Input: dimensioned drawing with shaded views. Units: mm. Origin: part minimum x, y, z. Give positions to 0.01 mm unless a question says otherwise; leave off trailing zeros. Loops run counter-clockwise (first coordinate to the right, second up) from the corner with the lowest first, then second, coordinate; pieces in that order, holes last.
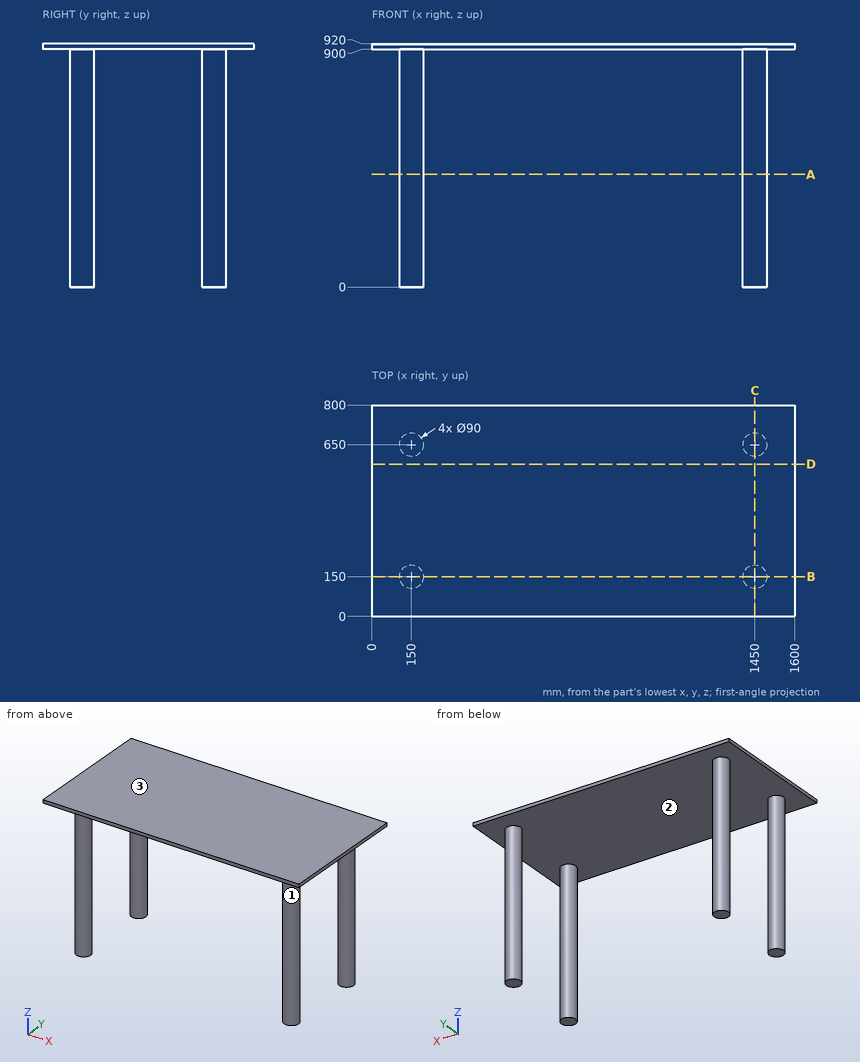
Item 1: Section query D-D on y = 576. Return loops of the section in (x, z), plus the area to 3 significant figures.
Values follow:
outline: (0, 900) - (1600, 900) - (1600, 920) - (0, 920) - close
area: 32,000 mm2
Item 2: Pin query (flat end, axial travel): pin 1 (5 mm diameter, centred on x = 468.5, y = 608.5, fed in from -Z). Return the tip coordinate at first contact, or that it passes through.
Values follow:
pin 1: stops at z = 900
Item 3: Section query B-B on y = 150. Return loops of the section in (x, z).
Values follow:
outline: (0, 900) - (105, 900) - (105, 0) - (195, 0) - (195, 900) - (1405, 900) - (1405, 0) - (1495, 0) - (1495, 900) - (1600, 900) - (1600, 920) - (0, 920) - close
Item 4: Ray query, probe 1 along Z at (x, y) = (194.5, 252.5); probe 2 along Y at (x, z) = (122.5, 771.5); probe 3 along X at (y, z) = (176.5, 828). Return the intervals inside material, ascending.
Values follow:
probe 1: z = 900 to 920
probe 2: y = 114.38 to 185.62, 614.38 to 685.62
probe 3: x = 113.63 to 186.37, 1413.63 to 1486.37
Item 5: Section query C-C on x = 1450. Return loops of the section in (y, z), plus the area to 3 significant figures.
Values follow:
outline: (0, 900) - (105, 900) - (105, 0) - (195, 0) - (195, 900) - (605, 900) - (605, 0) - (695, 0) - (695, 900) - (800, 900) - (800, 920) - (0, 920) - close
area: 178,000 mm2
Item 6: Draft query along X for the marked faces 1, 2 and 3. Return one class per face: +X half, -X half, draft (parallel to the pull), parting line (faces both ways), or undercut.
Values follow:
face 1: undercut
face 2: undercut
face 3: draft
Item 7: Section query A-A on z = 426.5. Return loops of the section in (x, y).
Values follow:
outline: circle Ø90 at (150, 150); circle Ø90 at (150, 650); circle Ø90 at (1450, 150); circle Ø90 at (1450, 650)
